Source: CAD feature listing. Evaluate the final solid. Frame: model axes, mm. Face numbers are marked on the shaded views. A direction names the side the tool comes from. Coordinates: 2 decimals unless noted, no trailing zeros. Loops run counter-clockwise (first coordinate to the right, second up) from the corner with the lowest first, then second, coordinate; pieces in that order, holes last. Notation, with made-up numbers: (73.5, 61) -> (118.5, 61) arc R12 ccw to (118.5, 78) -> close; hole circle Ø8 at (50.25, 36). An arc over 180 degrees is marked (long way). Answer as a JSON object with one key per item and string values. Group by question number.
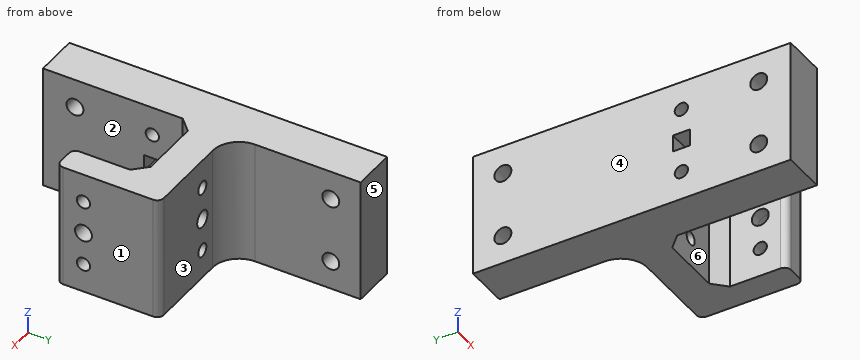
from build123d import *

# Parameters (mm, degrees)
BOSS_EXTRUDE1_DEPTH      = 23.8125
BOSS_EXTRUDE1_DEPTH_BACK = 23.8125
CUT_EXTRUDE1_DEPTH       = 41.213151732
CUT_EXTRUDE1_DEPTH_BACK  = 41.213151732
SKETCH6_R                = 2.5527
SKETCH6_R_2              = 3.2639
SKETCH7_R                = 1.5875
SKETCH7_W                = 6.5278
SKETCH7_H                = 6.5278
CUT_EXTRUDE2_DEPTH       = 41.213151732
SKETCH8_R                = 2.5527
CUT_EXTRUDE3_DEPTH       = 6.35
SKETCH14_R               = 3.2639
CUT_EXTRUDE6_DEPTH       = 46.858039931
SKETCH15_W               = 47.625
SKETCH15_H               = 33.3248
SKETCH15_R               = 2.5527
SKETCH15_W_2             = 6.5278
SKETCH15_H_2             = 6.5278
BOSS_EXTRUDE2_DEPTH      = 6.35
BOSS_EXTRUDE3_START      = 6.35
SKETCH16_W               = 47.625
SKETCH16_H               = 33.3248
SKETCH16_R               = 2.5527
SKETCH16_R_2             = 3.2639
BOSS_EXTRUDE3_DEPTH      = 6.35
BOSS_EXTRUDE4_START      = 6.35
SKETCH17_W               = 53.9496
SKETCH17_H               = 47.625
SKETCH17_R               = 2.5527
SKETCH17_R_2             = 3.2639
BOSS_EXTRUDE4_DEPTH      = 6.35
BOSS_EXTRUDE5_DEPTH      = 6.35
BOSS_EXTRUDE5_DEPTH_BACK = 10.31875
SKETCH19_R               = 2.5527
SKETCH19_W               = 6.5278
SKETCH19_H               = 6.5278
FILLET2_R                = 10.16
FILLET3_R                = 2.54
SKETCH20_R               = 3.2639
CUT_EXTRUDE7_DEPTH       = 93.145886885


with BuildPart() as part:
    # Sketch4 → Boss-Extrude1 (new, two sides: drawn at the far end of the back side and taken through both)
    with BuildSketch(Plane.XY.offset(-BOSS_EXTRUDE1_DEPTH_BACK)):
        Polygon((-20.6248, -24.9936), (-16.65605, -24.9936), (-16.65605, -2.9797375), (-11.6951125, 1.9812), (11.6951125, 1.9812), (16.65605, -2.9797375), (16.65605, -24.9936), (20.6248, -24.9936), (20.6248, 8.3312), (-20.6248, 8.3312), align=None)
    extrude(amount=BOSS_EXTRUDE1_DEPTH + BOSS_EXTRUDE1_DEPTH_BACK)

    # Sketch6 → Cut-Extrude1 (cut, two sides: drawn at the far end of the back side and taken through both)
    with BuildSketch(Plane(origin=(0, 0, 0), x_dir=(0, 0, -1), z_dir=(1, 0, 0)).offset(-CUT_EXTRUDE1_DEPTH_BACK)):
        with Locations((-12.7, -14.6812)):
            Circle(SKETCH6_R)
        with Locations((0, -14.6812)):
            Circle(SKETCH6_R_2)
        with Locations((12.7, -14.6812)):
            Circle(SKETCH6_R)
        with Locations((12.7, 16.6624)):
            Circle(SKETCH6_R_2)
        with Locations((-12.7, 16.6624)):
            Circle(SKETCH6_R_2)
    extrude(amount=CUT_EXTRUDE1_DEPTH + CUT_EXTRUDE1_DEPTH_BACK, mode=Mode.SUBTRACT)

    # Sketch7 → Cut-Extrude2 (cut, through all)
    with BuildSketch(Plane(origin=(0, 0, 0), x_dir=(0, 0, -1), z_dir=(1, 0, 0))):
        with Locations((-12.7, -14.6812)):
            Circle(SKETCH7_R)
        with Locations((12.7, -14.6812)):
            Circle(SKETCH7_R)
        with Locations((0, -14.6812)):
            Rectangle(SKETCH7_W, SKETCH7_H)
    extrude(amount=-CUT_EXTRUDE2_DEPTH, mode=Mode.SUBTRACT)

    # Sketch8 → Cut-Extrude3 (cut)
    with BuildSketch(Plane(origin=(0, 8.3312, 0), x_dir=(1, 0, 0), z_dir=(0, 1, 0))):
        with Locations(Location((0, 12.7, 0), (0, 0, 180))):
            Circle(SKETCH8_R)
        with Locations(Location((0, -12.7, 0), (0, 0, 180))):
            Circle(SKETCH8_R)
    extrude(amount=-CUT_EXTRUDE3_DEPTH, mode=Mode.SUBTRACT)

    # Sketch14 → Cut-Extrude6 (cut, through all)
    with BuildSketch(Plane(origin=(0, 8.3312, 0), x_dir=(1, 0, 0), z_dir=(0, 1, 0))):
        with Locations(Location((0, 0, 0), (0, 0, 180))):
            Circle(SKETCH14_R)
    extrude(amount=-CUT_EXTRUDE6_DEPTH, mode=Mode.SUBTRACT)

    # Sketch15 → Boss-Extrude2 (add)
    with BuildSketch(Plane.ZY.offset(20.6248)):
        with Locations((0, -8.3312)):
            Rectangle(SKETCH15_W, SKETCH15_H)
        with Locations(Location((12.7, -14.6812, 0), (0, 0, 180))):
            Circle(SKETCH15_R, mode=Mode.SUBTRACT)
        with Locations(Location((-12.7, -14.6812, 0), (0, 0, 180))):
            Circle(SKETCH15_R, mode=Mode.SUBTRACT)
        with Locations((0, -14.6812)):
            Rectangle(SKETCH15_W_2, SKETCH15_H_2, mode=Mode.SUBTRACT)
    extrude(amount=BOSS_EXTRUDE2_DEPTH)

    # Sketch16 → Boss-Extrude3 (add)
    with BuildSketch(Plane(origin=(20.6248, 0, 0), x_dir=(0, 0, -1), z_dir=(1, 0, 0)).offset(BOSS_EXTRUDE3_START)):
        with Locations((0, -8.3312)):
            Rectangle(SKETCH16_W, SKETCH16_H)
        with Locations((-12.7, -14.6812)):
            Circle(SKETCH16_R, mode=Mode.SUBTRACT)
        with Locations((0, -14.6812)):
            Circle(SKETCH16_R_2, mode=Mode.SUBTRACT)
        with Locations((12.7, -14.6812)):
            Circle(SKETCH16_R, mode=Mode.SUBTRACT)
    extrude(amount=-BOSS_EXTRUDE3_DEPTH)

    # Sketch17 → Boss-Extrude4 (add)
    with BuildSketch(Plane(origin=(0, 8.3312, 0), x_dir=(1, 0, 0), z_dir=(0, 1, 0)).offset(BOSS_EXTRUDE4_START)):
        Rectangle(SKETCH17_W, SKETCH17_H)
        with Locations(Location((0, -12.7, 0), (0, 0, 180))):
            Circle(SKETCH17_R, mode=Mode.SUBTRACT)
        with Locations(Location((0, 12.7, 0), (0, 0, 180))):
            Circle(SKETCH17_R, mode=Mode.SUBTRACT)
        with Locations(Location((0, 0, 0), (0, 0, 180))):
            Circle(SKETCH17_R_2, mode=Mode.SUBTRACT)
    extrude(amount=-BOSS_EXTRUDE4_DEPTH)

    # Sketch19 → Boss-Extrude5 (add, two sides: drawn at the far end of the back side and taken through both)
    with BuildSketch(Plane.ZY.offset(26.9748).offset(-BOSS_EXTRUDE5_DEPTH_BACK)):
        Polygon((-23.8125, 14.6812), (-23.8125, 65.4812), (23.8125, 65.4812), (23.8125, 14.6812), (23.8125, -24.9936), (23.8125, -56.7436), (-23.8125, -56.7436), (-23.8125, -24.9936), align=None)
        with Locations(Location((12.7, -14.6812, 0), (0, 0, 180))):
            Circle(SKETCH19_R, mode=Mode.SUBTRACT)
        with Locations(Location((-12.7, -14.6812, 0), (0, 0, 180))):
            Circle(SKETCH19_R, mode=Mode.SUBTRACT)
        with Locations((0, -14.6812)):
            Rectangle(SKETCH19_W, SKETCH19_H, mode=Mode.SUBTRACT)
    extrude(amount=BOSS_EXTRUDE5_DEPTH + BOSS_EXTRUDE5_DEPTH_BACK)

    # Fillet2
    fillet2_edges = [part.edges().sort_by_distance(p)[0] for p in [
        (-16.65605, 14.6812, 0),
    ]]
    fillet(fillet2_edges, radius=FILLET2_R)

    # Fillet3
    fillet3_edges = [part.edges().sort_by_distance(p)[0] for p in [
        (16.65605, -24.9936, 0),
        (26.9748, -24.9936, 0),
        (26.9748, 14.6812, 0),
    ]]
    fillet(fillet3_edges, radius=FILLET3_R)

    # Sketch20 → Cut-Extrude7 (cut, through all)
    with BuildSketch(Plane.ZY.offset(33.3248)):
        with Locations((-12.7, 53.975)):
            Circle(SKETCH20_R)
        with Locations((-12.7, -44.45)):
            Circle(SKETCH20_R)
        with Locations((12.7, 53.975)):
            Circle(SKETCH20_R)
        with Locations((12.7, -44.45)):
            Circle(SKETCH20_R)
    extrude(amount=-CUT_EXTRUDE7_DEPTH, mode=Mode.SUBTRACT)


solid = part.part
1. Section query D-D on x = -28. State how many separate pieces and enclosed holes the cut face has, then the cut area to 3 significant figures.
2. Section query A-A on y = -44.45. Return loops of the section in (x, z).
3. Mould query, pull axis X, two halves, no side actions, for the marked faces 4, 5 and 6. Classes: pulls with the +X half, pulls with the -X half, needs draft (parallel to the pull), parting line crosses it, or undercut.
4. Pin query (flat end, axial travel): pin 1 Ø8 at (x, z) = (0, -12.7) entering from +Y; pin 2 Ø8 at (x, z) = (-8, -7.5) entering from +Y; pin 3 Ø1.5 at (y, z) = (-33.5, -12) entering from +X. Return the tip coordinate at first contact, or that it passes through.
5. Reachability of the marked faces 1, 2 and 3 from +Z, -Z, +X, -X, +Y, -Y: full face, straight path, thin tool, end or side. Return the list, or none.
6. Section query B-B on x = 0. Return loops of the section in (y, z).
7. Section query C-C on z = 0. Return loops of the section in (x, y), then the cut area to 3 significant figures.
8. Ray query, L1, parallel to X at y = -18.5, z = 12; L2, parallel to Y at x = -26.5, z = -0.5; L3, parallel to Z at x = -24, y = -42. Return the intervals inside material, ascending.
Solved:
{
 "1": {"separate pieces": "1", "enclosed holes": "7", "area": "5,600 mm^2"},
 "2": {"outline": "(-33.32, -23.81) -> (-16.66, -23.81) -> (-16.66, -15.96) -> (-33.32, -15.96) -> close; (-33.32, -9.44) -> (-16.66, -9.44) -> (-16.66, 9.44) -> (-33.32, 9.44) -> close; (-33.32, 15.96) -> (-16.66, 15.96) -> (-16.66, 23.81) -> (-33.32, 23.81) -> close"},
 "3": {"face 4": "pulls with the -X half", "face 5": "needs draft", "face 6": "undercut"},
 "4": {"pin 1": "y = 14.68", "pin 2": "y = 16.3", "pin 3": "x = -16.66"},
 "5": {"face 1": "+Z, -Z, +X, +Y, -Y", "face 2": "+Z, -Z, -Y", "face 3": "+Z, -Z, +X, +Y"},
 "6": {"outline": "(1.98, -23.81) -> (14.68, -23.81) -> (14.68, -15.25) -> (1.98, -15.25) -> close; (1.98, -10.15) -> (14.68, -10.15) -> (14.68, -3.26) -> (1.98, -3.26) -> close; (1.98, 3.26) -> (14.68, 3.26) -> (14.68, 10.15) -> (1.98, 10.15) -> close; (1.98, 15.25) -> (14.68, 15.25) -> (14.68, 23.81) -> (1.98, 23.81) -> close"},
 "7": {"outline": "(-33.32, -56.74) -> (-16.66, -56.74) -> (-16.66, -17.95) -> (-33.32, -17.95) -> close; (-33.32, -11.42) -> (-16.66, -11.42) -> (-16.66, -2.98) -> (-11.7, 1.98) -> (-3.26, 1.98) -> (-3.26, 14.68) -> (-6.5, 14.68) arc R10.16 cw to (-16.66, 24.84) -> (-16.66, 65.48) -> (-33.32, 65.48) -> close; (3.26, 1.98) -> (11.7, 1.98) -> (16.66, -2.98) -> (16.66, -11.42) -> (26.97, -11.42) -> (26.97, 12.14) arc R2.54 ccw to (24.43, 14.68) -> (3.26, 14.68) -> close; (16.66, -22.45) arc R2.54 ccw to (19.2, -24.99) -> (24.43, -24.99) arc R2.54 ccw to (26.97, -22.45) -> (26.97, -17.95) -> (16.66, -17.95) -> close", "area": "2,650 mm^2"},
 "8": {"L1": "-33.32 to -16.66, 16.66 to 26.97", "L2": "-56.74 to -17.95, -11.42 to 65.48", "L3": "-23.81 to -14.86, -10.54 to 10.54, 14.86 to 23.81"}
}
